The model under review builds one solid part; all positions refer to its coordinate system, in mm. A direction names the side the tool comes from. Coordinates: 2 decimals unless noted, no trailing zeros. Order: outer loops, then holes, each group sorted by start corner. A loop starts at its lowest first (then second) coordinate and runs counter-clockwise, first axis right, second up. Notation, with made-up numbers: M 70.25,45.5 L 118.25,45.5 A13 cw 118.25,52.5 Z; hole C -15.5,-30.5 d4. An arc over 180 degrees is marked long. Answer as CSV lines item,"result". Start each with the question number.
Q1. Consider section A-A on z = -22. Write out the cut boundary in (x, y).
Q2. Consider section D-D on x = 34.5. Write out the cut boundary in (y, z), and give its area (3 significant figures).
Q3. The part is to be moulded in two halves that separate along X. For faces 6 (the face through (28.76, 12.32, -6.96)), 7 (the face through (27.005, 12.3, -23.6)), 8 (the face through (3, 0, -17)), 9 (the face through (-34.995, 12, -18)), say which applies: +X half, -X half, draft (parallel to the pull), parting line (faces both ways), or undercut.
Q4. Consider section C-C on z = -28. Write out the cut boundary in (x, y).
Q5. For P1, Ø5, axis at x = -17, y = 16, coming from the +Z side; P2, Ø7.5, axis at x = 0, y = 18, coming from the -Z side, all flat-tipped, find the tip position at first contact; note any pin that passes through.
Q6. Wall thickness on L1, parallel to Y at x = 32, z = -28; L2, parallel to X at y = 14.75, z = -21; L3, parallel to Z at x = -17, y = 18.75: over which ranges is each line inside the solid? List them lowest first. Write a range as [from, to].
Q7. Consider section B-B on y = 12.5. Write out the cut boundary in (x, z).
Q8. Machinability: for faces 1 (the face through (32.921, 16.466, -28.521)), 2 (the face through (2, 12, -10)), 3 (the face through (2, 12, -19)), 4 (the face through (-31, 12, -4)), 5 (the face through (3, 25, -17)), which of the approach directions +Z, -Z, +X, -X, +Y, -Y give a long, thin tool a straight path to every point of the face, cutting with its end or side? Answer none if there is none.
from build123d import *

# Parameters (mm, degrees)
BOSS_EXTRUDE1_DEPTH       = 25
F_8_0MM_DOWEL_HOLE2_D     = 8
F_8_0MM_DOWEL_HOLE2_DEPTH = 12


with BuildPart() as part:
    # Sketch1 → Boss-Extrude1 (new body)
    with BuildSketch(Plane(origin=(0, 0, 0), x_dir=(1, 0, 0), z_dir=(0, 1, 0))):
        Polygon((-34.995258132, 4), (-34.995258132, 33), (-33.263207324, 36), (-22.995258132, 36), (-22.995258132, 19), (27.004741868, 19), (27.004741868, 36), (39.004741868, 36), (39.004741868, 4), (30.468843483, 4), (27.004741868, 10), (-22.995258132, 10), (-26.459359747, 4), align=None)
    extrude(amount=BOSS_EXTRUDE1_DEPTH)

    # Ø8.0mm Dowel Hole2
    with Locations(Plane(origin=(39.004741868, 0, 0), x_dir=(0, 0, -1), z_dir=(1, 0, 0))):
        with Locations((28, 12.5)):
            Hole(F_8_0MM_DOWEL_HOLE2_D / 2, depth=F_8_0MM_DOWEL_HOLE2_DEPTH)


solid = part.part
Evaluation:
1,outline,"M -35,0 L -23,0 L -23,25 L -35,25 Z; M 27,0 L 39,0 L 39,25 L 27,25 Z"
2,outline,"M 0,-36 L 25,-36 L 25,-4 L 0,-4 Z; hole C 12.5,-28 d8"
2,area,"750 mm²"
3,face 6,"undercut"
3,face 7,"undercut"
3,face 8,"draft"
3,face 9,"-X half"
4,outline,"M -35,0 L -23,0 L -23,25 L -35,25 Z; M 27,0 L 39,0 L 39,8.5 L 27,8.5 Z; M 27,16.5 L 39,16.5 L 39,25 L 27,25 Z"
5,P1,"stops at z = -10"
5,P2,"stops at z = -19"
6,L1,"y = [0, 8.5], [16.5, 25]"
6,L2,"x = [-35, -23], [27, 39]"
6,L3,"z = [-19, -10]"
7,outline,"M -35,-33 L -33.26,-36 L -23,-36 L -23,-19 L 27,-19 L 27,-24 L 39,-24 L 39,-4 L 30.47,-4 L 27,-10 L -23,-10 L -26.46,-4 L -35,-4 Z; M 27,-36 L 39,-36 L 39,-32 L 27,-32 Z"
8,face 1,"+X"
8,face 2,"+Z, +Y, -Y"
8,face 3,"-Z, +Y, -Y"
8,face 4,"+Z, +X, -X, +Y, -Y"
8,face 5,"+Z, -Z, +X, -X, +Y"
